from build123d import *

# Parameters (mm, degrees)
F0_W     = 91.9
F0_H     = 156.9
F0_R     = 1.8
F1_DEPTH = 1
F2_R     = 3.25
F2_R_2   = 1.5
F3_DEPTH = 2


with BuildPart() as f1:
    # F0 (on Top) → F1 (new body)
    with BuildSketch(Plane.XY):
        Rectangle(F0_W, F0_H)
        with Locations((-41, -73.75)):
            Circle(F0_R, mode=Mode.SUBTRACT)
        with Locations((41, -73.75)):
            Circle(F0_R, mode=Mode.SUBTRACT)
        with Locations((-41, 73.75)):
            Circle(F0_R, mode=Mode.SUBTRACT)
        with Locations((41, 73.75)):
            Circle(F0_R, mode=Mode.SUBTRACT)
    extrude(amount=F1_DEPTH)

    # F2 (on face) → F3 (cut)
    with BuildSketch(Plane.XY.offset(1)):
        with Locations((20.9, 51.5)):
            Circle(F2_R)
        with Locations((-20.9, 51.5)):
            Circle(F2_R)
        with Locations((6.8, 51.5)):
            Circle(F2_R)
        with Locations((-6.8, 51.5)):
            Circle(F2_R)
        with BuildLine():
            Line((-37.5, -7.299998), (37.5, -7.299998))
            ThreePointArc((37.5, -7.299998), (37.853553, -7.153552), (38, -6.799998))
            Line((38, -6.799998), (38, 37.700002))
            ThreePointArc((38, 37.700002), (37.853553, 38.053555), (37.5, 38.200002))
            Line((37.5, 38.200002), (-37.5, 38.200002))
            ThreePointArc((-37.5, 38.200002), (-37.853553, 38.053555), (-38, 37.700002))
            Line((-38, 37.700002), (-38, -6.799998))
            ThreePointArc((-38, -6.799998), (-37.853553, -7.153552), (-37.5, -7.299998))
        make_face()
        with Locations((0, -19.799998)):
            Circle(F2_R_2)
        with Locations((0, -49.799998)):
            Circle(F2_R_2)
    extrude(amount=-F3_DEPTH, mode=Mode.SUBTRACT)


solid = f1.part
Geometry check sheet. Reference: the model listing, model coordinates, mm. Give positions to 0.01 mm unless a question says otherwise; leave off trailing zeros. Write each loop counter-clockwise with the first axis right and the second up, starting at its lowest first coordinate (ties: lowest second). Pieces come first, ordered by that corner, then holes. Notation, with made-up numbers: M 17,40.25 L 65,40.25 A16 ccw 65,70.25 Z; hole C 65,-39 d11. An arc over 180 degrees is marked long. One line per question, with ' | ' between items.
1. Gauge pin test, flat end, axial feed: pin 1 (1.8 mm diameter, centred on x = 0, y = -49.8, fed in from -Z). Record the tip position at first contact, or that the pin passes through.
Ans:
pin 1: through
2. Cross-section at B-B (x = -29.5). Enter the section's corners in (y, z), plus the area to 3 significant figures.
Ans:
outline: M -78.45,0 L -7.3,0 L -7.3,1 L -78.45,1 Z; M 38.2,0 L 78.45,0 L 78.45,1 L 38.2,1 Z | area: 111 mm2
3. Cross-section at D-D (x = 41). Enter the section's corners in (y, z), plus the area to 3 significant figures.
Ans:
outline: M -78.45,0 L -75.55,0 L -75.55,1 L -78.45,1 Z; M -71.95,0 L 71.95,0 L 71.95,1 L -71.95,1 Z; M 75.55,0 L 78.45,0 L 78.45,1 L 75.55,1 Z | area: 150 mm2
4. Cross-section at C-C (y = 51.5). Enter the section's corners in (x, z).
Ans:
outline: M -45.95,0 L -24.15,0 L -24.15,1 L -45.95,1 Z; M -17.65,0 L -10.05,0 L -10.05,1 L -17.65,1 Z; M -3.55,0 L 3.55,0 L 3.55,1 L -3.55,1 Z; M 10.05,0 L 17.65,0 L 17.65,1 L 10.05,1 Z; M 24.15,0 L 45.95,0 L 45.95,1 L 24.15,1 Z
5. Cross-section at A-A (y = -73.75). Enter the section's corners in (x, z), plus the area to 3 significant figures.
Ans:
outline: M -45.95,0 L -42.8,0 L -42.8,1 L -45.95,1 Z; M -39.2,0 L 39.2,0 L 39.2,1 L -39.2,1 Z; M 42.8,0 L 45.95,0 L 45.95,1 L 42.8,1 Z | area: 84.7 mm2
6. Scan lines: line 1 along Y through (x, z) = (20.9, 0.7); line 2 along X through (y, z) = (-73.75, 0.75); line 3 along Y through (x, z) = (41, 0.5). Record each from-to range of solid material in increasing order. Write a range as from..to.
Ans:
line 1: -78.45..-7.3, 38.2..48.25, 54.75..78.45 | line 2: -45.95..-42.8, -39.2..39.2, 42.8..45.95 | line 3: -78.45..-75.55, -71.95..71.95, 75.55..78.45
